Autodesk Inventor part; units mm, degrees
ref_plane "YZ Plane" through (0, 0, 0) normal (1, 0, 0) x (0, 1, 0)
ref_plane "XZ Plane" through (0, 0, 0) normal (0, 1, 0) x (-1, 0, 0)
ref_plane "XY Plane" through (0, 0, 0) normal (0, 0, 1) x (1, 0, 0)
sketch "Sketch1" plane through (0, 0, 0) normal (0, 1, 0) x (-1, 0, 0)
  line L0 (0, 0) -> (25.4, 0)
  line L1 (25.4, 0) -> (25.4, -25.4)
  line L2 (25.4, -25.4) -> (0, -25.4)
  line L3 (0, -25.4) -> (0, 0)
  line L4 (22.225, -22.225) -> (22.225, -3.175)
  line L5 (22.225, -3.175) -> (3.175, -3.175)
  line L6 (3.175, -3.175) -> (3.175, -22.225)
  line L7 (3.175, -22.225) -> (22.225, -22.225)
  dimension "d0" = 25.4
  dimension "d1" = 25.4
  dimension "d2" = 3.175
extrude "Extrusion1" add sketch "Sketch1" along normal blind 476.25
sketch "Sketch2" plane through (0, 0, 0) normal (1, 0, 0) x (0, 0, -1)
  line L0 (0, 0) -> (0, 476.25)
  line L1 (25.4, 0) -> (0, 0)
  line L2 (0, 476.25) -> (25.4, 476.25)
  point P0 (12.7, 50.8)
  point P1 (12.7, 425.45)
  dimension "d6" = 12.7
  dimension "d9" = 12.7
  dimension "d10" = 50.8
  dimension "d12" = 50.8
hole "Hole1" at (0, 50.8, -12.7) at (0, 425.45, -12.7) direction (-1, 0, 0) diameter 6.35 end through all
sketch "Sketch3" plane through (0, 0, -25.4) normal (0, 0, -1) x (-1, 0, 0)
  line L0 (25.4, 0) -> (0, 0)
  line L1 (0, 476.25) -> (25.4, 476.25)
  line L2 (25.4, 0) -> (25.4, 476.25)
  point P0 (9.525, 50.8)
  point P1 (9.525, 425.45)
  point P2 (9.525, 400.05)
  point P3 (9.525, 76.2)
  dimension "d20" = 50.8
  dimension "d21" = 50.8
  dimension "d22" = 25.4
  dimension "d23" = 25.4
  dimension "d24" = 15.875
  dimension "d25" = 15.875
  dimension "d26" = 15.875
  dimension "d27" = 15.875
hole "Hole2" at (-9.525, 50.8, -25.4) at (-9.525, 425.45, -25.4) at (-9.525, 400.05, -25.4) at (-9.525, 76.2, -25.4) direction (0, 0, 1) diameter 6.7469 end through all
properties part number "15102898-16-P-0209" material "Aluminum 6061"
Read the model definition and answer for the solid it produces. Units are mm, in the model's axes. A direction names the side the tool comes from. Round coordinates to 2 decimals unless told otherwise and drop trailing zeros. Order: outer loops, then holes, each group sorted by start corner. A loop starts at its lowest first (then second) coordinate and runs counter-clockwise, first axis right, second up.
1) The mould has two halves that part along Z. Classify faces 3 (the face through (-24, 0, -13)), 4 (the face through (-13, 235, -22.225)), 5 (the face through (-13, 235, 0)): released by +Z, released by -Z, zero draft, split by the parting line, or undercut.
2) A flat-ended cylindrical pin translates along its axis: pin 1 (4 mm diameter, centred on x = -9.525, y = 50.8, fed in from -Z). Find the tip coordinate at first contact, or state that the pin passes through.
3) Straight lines are drawn through the part: L1, parallel to Y at x = -24.2, z = -12.7 (3 decimals); L2, parallel to X at y = 357, z = -5 (3 decimals). For each, find the intervals that lie inside material, in ascending order.
4) The part is cut by section B-B on x = -18.25. Write down the section's boundary in (y, z) (3 decimals), plus the area to 3 significant figures.
5) For faces 1 (the face through (-22.225, 235, -13)), 2 (the face through (0, 235, -13)), determine the directions among +Z, -Z, +X, -X, +Y, -Y from which every point of the face is accessible in a straight line to the end or side of a thin tool.
6) The part is cut by section A-A on y = 35. Write down the section's boundary in (x, z) (3 decimals), plus the area to 3 significant figures.
Resolved:
1. face 3: zero draft
1. face 4: undercut
1. face 5: released by +Z
2. pin 1: passes through
3. L1: y = 0 to 47.625, 53.975 to 422.275, 428.625 to 476.25
3. L2: x = -25.4 to -22.225, -3.175 to 0
4. outline: (0, -25.4) - (476.25, -25.4) - (476.25, -22.225) - (0, -22.225) - close; (0, -3.175) - (476.25, -3.175) - (476.25, 0) - (0, 0) - close
4. area: 3,020 mm2
5. face 1: +Y, -Y
5. face 2: +Z, -Z, +X, +Y, -Y
6. outline: (-25.4, -25.4) - (0, -25.4) - (0, 0) - (-25.4, 0) - close; hole (-22.225, -22.225) - (-3.175, -22.225) - (-3.175, -3.175) - (-22.225, -3.175) - close
6. area: 282 mm2
